For this review, take the finished solid that the model builds, in its own axes (mm). A direction names the side the tool comes from. Give positions to 0.01 mm unless a question says otherwise; leave off trailing zeros. Write each loop counter-clockwise with the first axis right and the second up, starting at its lowest first coordinate (ties: lowest second). Pieces come first, ordered by that corner, then holes. Notation, with made-up numbers: (35.5, 50.5) -> (70.5, 50.5) arc R16 ccw to (70.5, 70.5) -> close; hole circle Ø1 at (75.25, -39). An arc over 180 degrees is marked (long way). Return JSON: item names as keys, results as strings.
from build123d import *

# Parameters (mm, degrees)
BOSS_EXTRUDE1_DEPTH = 12.7
CUT_EXTRUDE1_REACH  = 14.7
SKETCH1_R           = 2.60985
CUT_EXTRUDE2_REACH  = 14.7
SKETCH3_R           = 16.256
SKETCH5_R           = 2.0193
CUT_EXTRUDE3_DEPTH  = 12.7


with BuildPart() as part:
    # Sketch2 → Boss-Extrude1 (new body)
    with BuildSketch(Plane(origin=(0, 0, 0), x_dir=(1, 0, 0), z_dir=(0, 1, 0))):
        Polygon((-27.5, 0), (-27.5, 38.1), (27.5, 38.1), (27.5, 0), (27.5, -27.5), (-27.5, -27.5), align=None)
    extrude(amount=BOSS_EXTRUDE1_DEPTH)

    # Sketch1 → Cut-Extrude1 (cut, up to next)
    with BuildSketch(Plane(origin=(0, 0, 0), x_dir=(1, 0, 0), z_dir=(0, 1, 0)), mode=Mode.PRIVATE) as cut_extrude1_sk1:
        with Locations((15.909902577, 15.909902577)):
            Circle(SKETCH1_R)
    cut_extrude1_tool1 = extrude(cut_extrude1_sk1.sketch, amount=CUT_EXTRUDE1_REACH, mode=Mode.PRIVATE) & part.part
    add(cut_extrude1_tool1.solids().sort_by_distance((15.909903, 0, -15.909903))[0], mode=Mode.SUBTRACT)
    # Sketch1 → Cut-Extrude1 (cut, up to next)
    with BuildSketch(Plane(origin=(0, 0, 0), x_dir=(1, 0, 0), z_dir=(0, 1, 0)), mode=Mode.PRIVATE) as cut_extrude1_sk2:
        with Locations((-15.909902577, 15.909902577)):
            Circle(SKETCH1_R)
    cut_extrude1_tool2 = extrude(cut_extrude1_sk2.sketch, amount=CUT_EXTRUDE1_REACH, mode=Mode.PRIVATE) & part.part
    add(cut_extrude1_tool2.solids().sort_by_distance((-15.909903, 0, -15.909903))[0], mode=Mode.SUBTRACT)
    # Sketch1 → Cut-Extrude1 (cut, up to next)
    with BuildSketch(Plane(origin=(0, 0, 0), x_dir=(1, 0, 0), z_dir=(0, 1, 0)), mode=Mode.PRIVATE) as cut_extrude1_sk3:
        with Locations((15.909902577, -15.909902577)):
            Circle(SKETCH1_R)
    cut_extrude1_tool3 = extrude(cut_extrude1_sk3.sketch, amount=CUT_EXTRUDE1_REACH, mode=Mode.PRIVATE) & part.part
    add(cut_extrude1_tool3.solids().sort_by_distance((15.909903, 0, 15.909903))[0], mode=Mode.SUBTRACT)
    # Sketch1 → Cut-Extrude1 (cut, up to next)
    with BuildSketch(Plane(origin=(0, 0, 0), x_dir=(1, 0, 0), z_dir=(0, 1, 0)), mode=Mode.PRIVATE) as cut_extrude1_sk4:
        with Locations((-15.909902577, -15.909902577)):
            Circle(SKETCH1_R)
    cut_extrude1_tool4 = extrude(cut_extrude1_sk4.sketch, amount=CUT_EXTRUDE1_REACH, mode=Mode.PRIVATE) & part.part
    add(cut_extrude1_tool4.solids().sort_by_distance((-15.909903, 0, 15.909903))[0], mode=Mode.SUBTRACT)

    # Sketch3 → Cut-Extrude2 (cut, up to next)
    with BuildSketch(Plane.XZ, mode=Mode.PRIVATE) as cut_extrude2_sk1:
        Circle(SKETCH3_R)
    cut_extrude2_tool1 = extrude(cut_extrude2_sk1.sketch, amount=-CUT_EXTRUDE2_REACH, mode=Mode.PRIVATE) & part.part
    add(cut_extrude2_tool1.solids().sort_by_distance((0, 0, 0))[0], mode=Mode.SUBTRACT)

    # Sketch5 → Cut-Extrude3 (cut)
    with BuildSketch(Plane(origin=(0, 0, -38.1), x_dir=(-1, 0, 0), z_dir=(0, 0, -1))):
        with Locations((6.35, 6.35)):
            Circle(SKETCH5_R)
        with Locations((19.05, 6.35)):
            Circle(SKETCH5_R)
        with Locations((-19.05, 6.35)):
            Circle(SKETCH5_R)
        with Locations((-6.35, 6.35)):
            Circle(SKETCH5_R)
    extrude(amount=-CUT_EXTRUDE3_DEPTH, mode=Mode.SUBTRACT)


solid = part.part
1. The part is to be moulded in two halves that separate along Z. For faces 1 (the cylindrical face through (-3.52, 6.26, -15.87)), 2 (the cylindrical face through (4.485, 5.577, -31.839)), 3 (the flat face through (19, 6, -25.4)), 4 (the cylindrical face through (-17.833, 6.261, 14.146)), say which applies: +Z half, -Z half, draft (parallel to the pull), parting line (faces both ways), or undercut.
Results found:
{"face 1": "undercut", "face 2": "draft", "face 3": "-Z half", "face 4": "undercut"}
2. To check wall thickness, follow probe 1 along Y at (x, z) = (19, -30); probe 2 along Z at (x, y) = (14, 2.75); probe 3 along X at (y, z) = (11, 15). State the ranges of each line that lie inside material, in increasing order.
Results found:
{"probe 1": "y = 0 to 4.33, 8.37 to 12.7", "probe 2": "z = -38.1 to -17.69, -14.13 to -8.26, 8.26 to 14.13, 17.69 to 27.5", "probe 3": "x = -27.5 to -18.36, -13.46 to -6.27, 6.27 to 13.46, 18.36 to 27.5"}
3. Add section D-D, the plane z = 1.5. State the section outline as (x, y) points.
Results found:
{"outline": "(-27.5, 0) -> (-16.19, 0) -> (-16.19, 12.7) -> (-27.5, 12.7) -> close; (16.19, 0) -> (27.5, 0) -> (27.5, 12.7) -> (16.19, 12.7) -> close"}
4. Add section A-A, the plane z = -28. State the section outline as (x, y) points.
Results found:
{"outline": "(-27.5, 0) -> (27.5, 0) -> (27.5, 12.7) -> (-27.5, 12.7) -> close; hole circle Ø4.04 at (-19.05, 6.35); hole circle Ø4.04 at (-6.35, 6.35); hole circle Ø4.04 at (6.35, 6.35); hole circle Ø4.04 at (19.05, 6.35)"}
5. For pin 1 (1.2 mm diameter, centred on x = -18.5, y = 6.5, fed in from -Z); pin 2 (4.5 mm diameter, centred on x = -15.91, z = -15.91, fed in from +Y), all flat-tipped, find the tip position at first contact; note any pin that passes through.
Results found:
{"pin 1": "stops at z = -25.4", "pin 2": "passes through"}
6. Add section C-C, the plane y = 5.5. State the section outline as (x, z) points.
Results found:
{"outline": "(-27.5, -38.1) -> (-20.88, -38.1) -> (-20.88, -25.4) -> (-17.22, -25.4) -> (-17.22, -38.1) -> (-8.18, -38.1) -> (-8.18, -25.4) -> (-4.52, -25.4) -> (-4.52, -38.1) -> (4.52, -38.1) -> (4.52, -25.4) -> (8.18, -25.4) -> (8.18, -38.1) -> (17.22, -38.1) -> (17.22, -25.4) -> (20.88, -25.4) -> (20.88, -38.1) -> (27.5, -38.1) -> (27.5, 27.5) -> (-27.5, 27.5) -> close; hole circle Ø5.22 at (-15.91, -15.91); hole circle Ø5.22 at (-15.91, 15.91); hole circle Ø32.51 at (0, 0); hole circle Ø5.22 at (15.91, -15.91); hole circle Ø5.22 at (15.91, 15.91)"}
7. Add section B-B, the plane x = 0. State the section outline as (y, z) points.
Results found:
{"outline": "(0, -38.1) -> (12.7, -38.1) -> (12.7, -16.26) -> (0, -16.26) -> close; (0, 16.26) -> (12.7, 16.26) -> (12.7, 27.5) -> (0, 27.5) -> close"}
8. For faces 5 (the flat face through (0, 6, -38.1)), 6 (the cylindrical face through (17.185, 5.577, -31.839)), list the 3-axis set-ups (+Z, -Z, +X, -X, +Y, -Y) from which the entire face can be reached by the end or side of a thin tool; tool diameter is ignored.
Results found:
{"face 5": "-Z, +X, -X, +Y, -Y", "face 6": "-Z"}
